```python
from build123d import *

# Parameters (mm, degrees)
SKETCH1_R           = 3
BOSS_EXTRUDE1_DEPTH = 2.54
SKETCH2_R           = 3
BOSS_EXTRUDE2_DEPTH = 2.54
SKETCH3_R           = 0.5
CUT_EXTRUDE1_DEPTH  = 10


with BuildPart() as part:
    # Sketch1 → Boss-Extrude1 (new body)
    with BuildSketch(Plane(origin=(0, 0, 0), x_dir=(1, 0, 0), z_dir=(0, 1, 0))):
        with Locations(Location((0, 0, 0), (0, 0, 270))):
            Circle(SKETCH1_R)
    extrude(amount=BOSS_EXTRUDE1_DEPTH)

    # Sketch2 → Boss-Extrude2 (add)
    with BuildSketch(Plane(origin=(0, 2.54, 0), x_dir=(1, 0, 0), z_dir=(0, 1, 0))):
        with BuildLine():
            ThreePointArc((-3, 15), (0, 18), (3, 15))
            Line((3, 15), (-3, 15))
        make_face()
        Polygon((-3, 15), (-3, 3), (0, 3), (3, 3), (3, 15), align=None)
        with BuildLine():
            Line((-5.08, 3), (-5.08, -3))
            ThreePointArc((-5.08, -3), (-8.08, 0), (-5.08, 3))
        make_face()
        Polygon((-3, 3), (-5.08, 3), (-5.08, -3), (-3, -3), (-3, 6e-09), align=None)
        with BuildLine():
            Line((3, 3), (0, 3))
            ThreePointArc((0, 3), (2.121320344, 2.121320344), (3, 0))
            Line((3, 0), (3, 3))
        make_face()
        with Locations(Location((0, 0, 0), (0, 0, 270))):
            Circle(SKETCH2_R)
        with BuildLine():
            Line((3, -3), (3, 0))
            ThreePointArc((3, 0), (2.121320338, -2.121320349), (-1.5e-08, -3))
            Line((-1.5e-08, -3), (3, -3))
        make_face()
        with BuildLine():
            ThreePointArc((5.08, 3), (8.08, 0), (5.08, -3))
            Line((5.08, -3), (5.08, 3))
        make_face()
        Polygon((5.08, 3), (3, 3), (3, 0), (3, -3), (5.08, -3), align=None)
        with BuildLine():
            ThreePointArc((-1.5e-08, -3), (-2.121320351, -2.121320336), (-3, 6e-09))
            Line((-3, 6e-09), (-3, -3))
            Line((-3, -3), (-1.5e-08, -3))
        make_face()
        with BuildLine():
            Line((0, 3), (-3, 3))
            Line((-3, 3), (-3, 6e-09))
            ThreePointArc((-3, 6e-09), (-2.121320342, 2.121320346), (0, 3))
        make_face()
    extrude(amount=BOSS_EXTRUDE2_DEPTH)

    # Sketch3 → Cut-Extrude1 (cut)
    with BuildSketch(Plane(origin=(0, 5.08, 0), x_dir=(1, 0, 0), z_dir=(0, 1, 0))):
        with Locations(Location((0, 16.5, 0), (0, 0, 270))):
            Circle(SKETCH3_R)
        with Locations(Location((0, 14.5, 0), (0, 0, 270))):
            Circle(SKETCH3_R)
        with Locations(Location((0, 12.5, 0), (0, 0, 270))):
            Circle(SKETCH3_R)
        with Locations(Location((0, 10.5, 0), (0, 0, 270))):
            Circle(SKETCH3_R)
        with Locations(Location((0, 8.5, 0), (0, 0, 270))):
            Circle(SKETCH3_R)
        with Locations(Location((0, 6.5, 0), (0, 0, 270))):
            Circle(SKETCH3_R)
        with Locations(Location((0, 4.5, 0), (0, 0, 270))):
            Circle(SKETCH3_R)
    extrude(amount=-CUT_EXTRUDE1_DEPTH, mode=Mode.SUBTRACT)


solid = part.part
```
For this review, take the finished solid that the model builds, in its own axes (mm). A direction names the side the tool comes from. Round coordinates to 2 decimals unless told otherwise and drop trailing zeros. Write each loop counter-clockwise with the first axis right and the second up, starting at its lowest first coordinate (ties: lowest second). Pieces come first, ordered by that corner, then holes. Notation, with made-up numbers: (59.5, 42.5) - (97.5, 42.5) arc R26 ccw to (97.5, 77.5) - close; hole circle Ø5 at (-24.75, 53). An arc over 180 degrees is marked (long way). Answer as a JSON object with one key per item and string values.
1. For pin 1 Ø0.6 at (x, y) = (-4, 3) entering from -Z; pin 2 Ø2 at (y, z) = (3.5, -7) entering from -X; pin 3 Ø5 at (x, z) = (-2, -11) entering from -Y, all flat-tipped, find the tip position at first contact; note any pin that passes through.
Response values:
{"pin 1": "stops at z = -3", "pin 2": "stops at x = -3", "pin 3": "stops at y = 2.54"}
2. We need section B-B on y = 3.45. Give the boundary of the cut face in (x, z).
Response values:
{"outline": "(-5.08, -3) - (-3, -3) - (-3, -15) arc R3 ccw to (3, -15) - (3, -3) - (5.08, -3) arc R3 ccw to (5.08, 3) - (-5.08, 3) arc R3 ccw to start; hole circle Ø1 at (0, -16.5); hole circle Ø1 at (0, -14.5); hole circle Ø1 at (0, -12.5); hole circle Ø1 at (0, -10.5); hole circle Ø1 at (0, -8.5); hole circle Ø1 at (0, -6.5); hole circle Ø1 at (0, -4.5)"}
3. To check wall thickness, follow line 1 along X through (y, z) = (3.9, -12.5); line 2 along X through (y, z) = (2.8, -8.75); line 3 along Z through (x, y) = (4.75, 3.8). State the ranges of each line that lie inside material, in increasing order.
Response values:
{"line 1": "x = -3 to -0.5, 0.5 to 3", "line 2": "x = -3 to -0.43, 0.43 to 3", "line 3": "z = -3 to 3"}
4. Tool access review of faces 1 (the face through (-3, 4, -9)), 2 (the face through (3, 4, -9)), 3 (the face through (0, 4, -13)): name each direction out of +Z, -Z, +X, -X, +Y, -Y from which nothing blocks a thin tool from reaching the whole face with its end or side.
Response values:
{"face 1": "-Z, -X, +Y, -Y", "face 2": "-Z, +X, +Y, -Y", "face 3": "+Y, -Y"}
5. We need section D-D on z = -9.75. Give the boundary of the cut face in (x, y), then the cut area to 3 significant figures.
Response values:
{"outline": "(-3, 2.54) - (3, 2.54) - (3, 5.08) - (-3, 5.08) - close", "area": "15.2 mm2"}
6. We need section A-A on z = -14.5. Give the boundary of the cut face in (x, y), then the cut area to 3 significant figures.
Response values:
{"outline": "(-3, 2.54) - (-0.5, 2.54) - (-0.5, 5.08) - (-3, 5.08) - close; (0.5, 2.54) - (3, 2.54) - (3, 5.08) - (0.5, 5.08) - close", "area": "12.7 mm2"}
7. Draft analysis for pull direction X (two halves, no side actions). For faces 4 (the face through (0.9, 1.25, 2.86)), 5 (the face through (0, 4, -5)), 6 (the face through (4, 4, -3)), state which applies: +X half, -X half, draft (parallel to the pull), parting line (faces both ways), or undercut.
Response values:
{"face 4": "parting line", "face 5": "undercut", "face 6": "draft"}
8. We need section C-C on x = -0.75. Give the boundary of the cut face in (y, z).
Response values:
{"outline": "(0, -2.9) - (2.54, -2.9) - (2.54, -17.9) - (5.08, -17.9) - (5.08, 3) - (2.54, 3) - (2.54, 2.9) - (0, 2.9) - close"}
